```python
from build123d import *

# Parameters (mm, degrees)
BOSS_EXTRU_1_DEPTH      = 2
ESQUISSE2_R             = 1.4
BOSS_EXTRU_2_DEPTH      = 2
ESQUISSE3_R             = 1.6
BOSS_EXTRU_3_DEPTH      = 1
ESQUISSE4_W             = 4
ESQUISSE4_H             = 1
ENL_V_MAT_EXTRU_1_DEPTH = 3


with BuildPart() as part:
    # Esquisse1 → Boss.-Extru.1 (new body)
    with BuildSketch(Plane.XY):
        with BuildLine():
            Line((-27.09345354, 2.075059053), (-32.253315255, -10.939387807))
            ThreePointArc((-32.253315255, -10.939387807), (-35.4987275, -12.341992297), (-36.901331991, -9.096580052))
            Line((-36.901331991, -9.096580052), (-31.741470275, 3.917866809))
            ThreePointArc((-31.741470275, 3.917866809), (-28.49605803, 5.320471299), (-27.09345354, 2.075059053))
        make_face()
    extrude(amount=BOSS_EXTRU_1_DEPTH)

    # Esquisse2 → Boss.-Extru.2 (add)
    with BuildSketch(Plane(origin=(0, 0, 0), x_dir=(-1, 0, 0), z_dir=(0, 0, -1))):
        with Locations(Location((29.417461908, 2.996462931, 0), (0, 0, 180))):
            Circle(ESQUISSE2_R)
        with Locations(Location((34.577323623, -10.017983929, 0), (0, 0, 180))):
            Circle(ESQUISSE2_R)
    extrude(amount=BOSS_EXTRU_2_DEPTH)

    # Esquisse3 → Boss.-Extru.3 (add)
    with BuildSketch(Plane(origin=(0, 0, -2), x_dir=(-1, 0, 0), z_dir=(0, 0, -1))):
        with Locations((34.577323623, -10.017983929)):
            Circle(ESQUISSE3_R)
        with Locations((29.417461908, 2.996462931)):
            Circle(ESQUISSE3_R)
    extrude(amount=BOSS_EXTRU_3_DEPTH)

    # Esquisse4 → Enlèv. mat.-Extru.1 (cut)
    with BuildSketch(Plane(origin=(0, 0, -3), x_dir=(-1, 0, 0), z_dir=(0, 0, -1))):
        with Locations((29.417461908, 2.996462931)):
            Rectangle(ESQUISSE4_W, ESQUISSE4_H)
        with Locations((34.577323623, -10.017983929)):
            Rectangle(ESQUISSE4_W, ESQUISSE4_H)
    extrude(amount=-ENL_V_MAT_EXTRU_1_DEPTH, mode=Mode.SUBTRACT)


solid = part.part
```
Geometry: final body of the model. Coordinates: model frame, mm. A direction names the side the tool comes from. Coordinates: 2 decimals unless noted, no trailing zeros. Write each loop counter-clockwise with the first axis right and the second up, starting at its lowest first coordinate (ties: lowest second). Pieces come first, ordered by that corner, then holes. Notation, with made-up numbers: M 57.5,64.25 L 80.5,64.25 A14 cw 80.5,89.25 Z; hole C 35,46.5 d1. An arc over 180 degrees is marked long. Use CSV: the item, a comma, the result in double quotes. Start each with the question number.
1. Cut plane D-D on z = 1.1. Return the cut outline in (x, y), plus the area to 3 significant figures.
2. Mould query, pull axis Z, two halves, no side actions, for faces 1 (the face through (-29.637, -4.341, 0.986)), 2 (the face through (-35, -11, -3)), 3 (the face through (-34.6, -8.62, -0.99)), 4 (the face through (-29.394, 1.597, -0.986)). Classes: pulls with the +Z half, pulls with the -Z half, needs draft (parallel to the pull), parting line crosses it, or undercut.
3. Ray query, probe 1 along Z at (x, y) = (-35.75, -11); probe 2 along Y at (x, z) = (-33.25, -2.5); probe 3 along Z at (x, y) = (-31.75, 0.5). Return the intervals inside material, ascending.
4. First-contact query: P1, Ø1, axis at y = -4, z = 0.5, coming from the +X side; P2, Ø1.5, axis at x = -29, z = -1, coming from the +Y side; P3, Ø1.5, axis at x = -34, z = -1, coming from the -Y side; P4, Ø5, axis at x = -31.5, y = -10.5, coming from the -Z side. Flat tips, straight axial feed; report the tip coordinate or a pass-through.
5. Reachability of faces 5 (the face through (-35, -9, -3)), 6 (the face through (-29, 3.496, -2)), 7 (the face through (-34.61, -8.42, -2.49)) from +Z, -Z, +X, -X, +Y, -Y: full face, straight path, thin tool, end or side. Return the list, or none.
6. Cut plane C-C on z = -0.5. Return the cut outline in (x, y) (3 decimals).
7. Cut plane A-A on z = -2.2. Return the cut outline in (x, y), plus the area to 3 significant figures.
8. Cut plane B-B on x = -29. Return the cut outline in (y, z), plus the area to 3 significant figures.
Entries:
1,outline,"M -36.9,-9.1 A2.5 ccw -32.25,-10.94 L -27.09,2.08 A2.5 ccw -31.74,3.92 Z"
1,area,"89.6 mm²"
2,face 1,"needs draft"
2,face 2,"pulls with the -Z half"
2,face 3,"undercut"
2,face 4,"undercut"
3,probe 1,"-3 to -2, 0 to 2"
3,probe 2,"-10.91 to -10.52, -9.52 to -9.12"
3,probe 3,"0 to 2"
4,P1,"x = -29.3"
4,P2,"y = 4.4"
4,P3,"y = -11.42"
4,P4,"z = -3"
5,face 5,"-Z, +X, -X, +Y, -Y"
5,face 6,"-Z, +X, -X"
5,face 7,"-Z, +Y"
6,outline,"M -35.885,-10.518 A1.4 ccw -33.27,-10.518 Z; M -35.885,-9.518 L -33.27,-9.518 A1.4 ccw Z; M -30.725,2.496 A1.4 ccw -28.11,2.496 Z; M -30.725,3.496 L -28.11,3.496 A1.4 ccw Z"
7,outline,"M -36.1,-10.52 A1.6 ccw -33.06,-10.52 Z; M -36.1,-9.52 L -33.06,-9.52 A1.6 ccw Z; M -30.94,2.5 A1.6 ccw -27.9,2.5 Z; M -30.94,3.5 L -27.9,3.5 A1.6 ccw Z"
7,area,"9.79 mm²"
8,outline,"M -2.73,0 L 1.66,0 L 1.66,-2 L 1.45,-2 L 1.45,-3 L 2.5,-3 L 2.5,0 L 3.5,0 L 3.5,-3 L 4.54,-3 L 4.54,-2 L 4.33,-2 L 4.33,0 L 5.46,0 L 5.46,2 L -2.73,2 Z"
8,area,"21.8 mm²"
